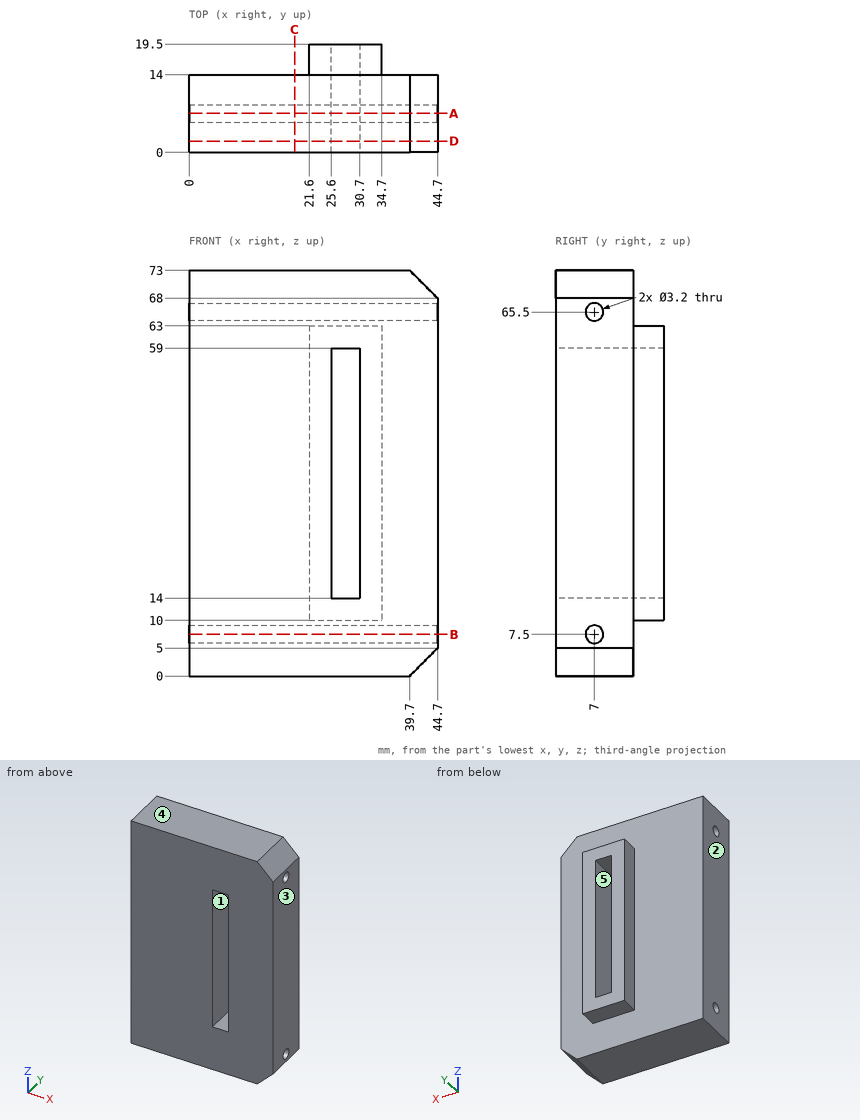
Drawing for the job (mm, zero at the part's lowest x, y, z). A direction names the side the tool comes from. Round coordinates to 2 decimals unless told otherwise and drop trailing zeros. Loops run counter-clockwise (first coordinate to the right, second up) from the corner with the lowest first, then second, coordinate; pieces in that order, holes last.
1. Band-saw the part on B-B, the plane z = 7.5. List the corners of the cut face in (x, y), and give its area (3 significant figures).
Check values:
outline: (0, 0) - (44.7, 0) - (44.7, 5.4) - (0, 5.4) - close; (0, 8.6) - (44.7, 8.6) - (44.7, 14) - (0, 14) - close
area: 483 mm2
2. Band-saw the part on C-C, the plane x = 19. List the corners of the cut face in (y, z), and give its area (3 significant figures).
Check values:
outline: (0, 0) - (14, 0) - (14, 73) - (0, 73) - close; hole circle Ø3.2 at (7, 7.5); hole circle Ø3.2 at (7, 65.5)
area: 1,010 mm2
3. Band-saw the part on D-D, the plane y = 2. List the corners of the cut face in (x, z).
Check values:
outline: (0, 0) - (39.7, 0) - (44.7, 5) - (44.7, 68) - (39.7, 73) - (0, 73) - close; hole (25.6, 14) - (30.7, 14) - (30.7, 59) - (25.6, 59) - close
4. Band-saw the part on A-A, the plane y = 7. List the corners of the cut face in (x, z), and give its area (3 significant figures).
Check values:
outline: (0, 0) - (39.7, 0) - (44.7, 5) - (44.7, 5.9) - (0, 5.9) - close; (0, 9.1) - (44.7, 9.1) - (44.7, 63.9) - (0, 63.9) - close; (0, 67.1) - (44.7, 67.1) - (44.7, 68) - (39.7, 73) - (0, 73) - close; hole (25.6, 14) - (30.7, 14) - (30.7, 59) - (25.6, 59) - close
area: 2,720 mm2
5. Tool access for the marked faces 4 and 5: list every direction of +Z, -Z, +X, -X, +Y, -Y with a clear straight run to the whole face (end or side of a thin tool).
Check values:
face 4: +Z, +X, -X, +Y, -Y
face 5: +Y, -Y
6. Wall check: probe 1 along Y at (x, z) = (35, 65.5); probe 2 along X at (y, z) = (5, 29); probe 3 along X at (y, z) = (15.25, 36.5). Give the ranges that are in metal, low to high.
Check values:
probe 1: y = 0 to 5.4, 8.6 to 14
probe 2: x = 0 to 25.6, 30.7 to 44.7
probe 3: x = 21.6 to 25.6, 30.7 to 34.7
7. Drop flat-ended pins along their axis: P1, Ø2.5, axis at x = 28.5, y = 17.5, coming from the -Z side; P2, Ø2, axis at x = 8.5, z = 19.5, coming from the +Y side; P3, Ø3, axis at y = 16, z = 35.5, coming from the +X side. Give the stop position or say it passes through.
Check values:
P1: stops at z = 10
P2: stops at y = 14
P3: stops at x = 34.7
8. Mould opens along X. For the marked faces 1, 2 and 3 say: +X half, -X half, draft (parallel to the pull), parting line (faces both ways), or undercut.
Check values:
face 1: undercut
face 2: -X half
face 3: +X half
